Geometry: final body of the model. Coordinates: model frame, mm. A direction names the side the tool comes from. Round coordinates to 2 decimals unless told otherwise and drop trailing zeros. Order: outer loops, then holes, each group sorted by start corner. A loop starts at its lowest first (then second) coordinate and runs counter-clockwise, first axis right, second up. Notation, with made-up numbers: (-5, 11) - (23, 11) arc R8 cw to (23, 17) - close; hole circle Ø4 at (3.5, 46.5). An arc over 180 degrees is marked (long way). Put each result on its own line as item: value. Start each with the question number.
(1) Section A-A (x = 10). Output: boundary loops of the cut face in (y, z), and give its area (3 significant figures).
(2) Material intervals for L1, parallel to Y at x = -8.75, z = 2; L2, parallel to Z at x = 7.25, y = -3, sorted ascending. Write a range as [from, to].
(3) Section B-B (z = 23.75). Output: boundary loops of the cut face in (x, y).
(4) Access query for faces 4 (the face through (0, 0, 28.4)), 5 (the face through (14.4, -14.43, 15.21)). Directions: +Z, -Z, +X, -X, +Y, -Y. A direction counts if a zero-diameter tool reaches every point of the face in a straight line with its end or side. Return the directions, or none.
(5) Pull-direction query (X, two-part tool) for faces 1 (the face through (0, -13.4, 15)), 2 (the face through (-14.43, -14.4, 15.21)), 3 (the face through (15, 0, 15)); classes: released by +X, released by -X, zero draft, split by the parting line, or undercut.
Autodesk Fusion 360 part; units mm, degrees
sketch "Sketch1" plane through (0, 0, 0) normal (0, 0, 1) x (1, 0, 0)
  line L0 (15, -15) -> (-15, -15)
  line L1 (-15, -15) -> (-15, 15)
  line L2 (-15, 15) -> (15, 15)
  line L3 (15, 15) -> (15, -15)
  line L4 (15, -15) -> (-15, 15) construction
  line L5 (-15, -15) -> (15, 15) construction
  dimension "d1" = 30
  dimension "d2" = 30
extrude "Extrude1" add sketch "Sketch1" along normal blind 30
fillet "Fillet1" radius 2 4 edges at (-15, -15, 15) (15, -15, 15) (15, 15, 15) (-15, 15, 15)
shell "Shell1" thickness 1.6 removed faces 1 at (4.3333, -5, 30)
sketch "Sketch2" plane through (0, 0, 30) normal (0, 0, 1) x (-1, 0, 0)
  arc A0 (-13.4, -13) -> (-13, -13.4) centre (-13, -13) ccw
  line L0 (-13.4, -13) -> (-13.4, 13)
  arc A1 (-13, 13.4) -> (-13.4, 13) centre (-13, 13) ccw
  line L1 (-13, 13.4) -> (13, 13.4)
  arc A2 (13.4, 13) -> (13, 13.4) centre (13, 13) ccw
  line L2 (13.4, 13) -> (13.4, -13)
  arc A3 (13, -13.4) -> (13.4, -13) centre (13, -13) ccw
  line L3 (13, -13.4) -> (-13, -13.4)
  arc A4 (13, -15) -> (15, -13) centre (13, -13) ccw
  line L4 (15, -13) -> (15, 13)
  arc A5 (15, 13) -> (13, 15) centre (13, 13) ccw
  line L5 (13, 15) -> (-13, 15)
  arc A6 (-13, 15) -> (-15, 13) centre (-13, 13) ccw
  line L6 (-15, 13) -> (-15, -13)
  arc A7 (-15, -13) -> (-13, -15) centre (-13, -13) ccw
  line L7 (-13, -15) -> (13, -15)
extrude "Extrude2" add sketch "Sketch2" against normal blind 1.6 contours A0 L0 A1 L1 A2 L2 A3 L3
Checks:
1. outline: (-15, 0) - (15, 0) - (15, 30) - (-15, 30) - close; hole (-13.4, 1.6) - (13.4, 1.6) - (13.4, 28.4) - (-13.4, 28.4) - close
1. area: 182 mm²
2. L1: y = [-15, -13.4], [13.4, 15]
2. L2: z = [0, 1.6], [28.4, 30]
3. outline: (-15, -13) arc R2 ccw to (-13, -15) - (13, -15) arc R2 ccw to (15, -13) - (15, 13) arc R2 ccw to (13, 15) - (-13, 15) arc R2 ccw to (-15, 13) - close; hole (-13.4, -13) arc R0.4 ccw to (-13, -13.4) - (13, -13.4) arc R0.4 ccw to (13.4, -13) - (13.4, 13) arc R0.4 ccw to (13, 13.4) - (-13, 13.4) arc R0.4 ccw to (-13.4, 13) - close
4. face 4: none
4. face 5: +Z, -Z, +X, -Y
5. face 1: undercut
5. face 2: released by -X
5. face 3: released by +X
